from build123d import *

# Parameters (mm, degrees)
SKETCH1_R                           = 14.2875
SKETCH1_R_2                         = 9.525
BOSS_EXTRUDE1_DEPTH                 = 304.8
SKETCH2_R                           = 11.1125
CUT_EXTRUDE1_DEPTH                  = 19.05
CUT_EXTRUDE4_DEPTH                  = 76.2
CUT_EXTRUDE7_DEPTH                  = 12.7
CUT_EXTRUDE8_REACH                  = 308.326
CUT_EXTRUDE8_END_RADIUS             = 9.525
CUT_EXTRUDE8_DIRECTION_2_REACH      = 308.326
CUT_EXTRUDE8_DIRECTION_2_END_RADIUS = 14.2875


with BuildPart() as part:
    # Sketch1 → Boss-Extrude1 (new body)
    with BuildSketch(Plane.XY):
        with Locations(Location((0, 0, 0), (0, 0, 180))):
            Circle(SKETCH1_R)
        with Locations(Location((0, 0, 0), (0, 0, 180))):
            Circle(SKETCH1_R_2, mode=Mode.SUBTRACT)
    extrude(amount=BOSS_EXTRUDE1_DEPTH)

    # Sketch2 → Cut-Extrude1 (cut)
    with BuildSketch(Plane.XY.offset(304.8)):
        Circle(SKETCH2_R)
    extrude(amount=-CUT_EXTRUDE1_DEPTH, mode=Mode.SUBTRACT)

    # Sketch6 → Cut-Extrude4 (cut)
    with BuildSketch(Plane(origin=(0, 0, 0), x_dir=(-1, 0, 0), z_dir=(0, 0, -1))):
        with BuildLine():
            Line((14.2875, 0), (-14.2875, 0))
            ThreePointArc((-14.2875, 0), (0, -14.2875), (14.2875, 0))
        make_face()
    extrude(amount=-CUT_EXTRUDE4_DEPTH, mode=Mode.SUBTRACT)

    # Sketch8 → Cut-Extrude7 (cut)
    with BuildSketch(Plane(origin=(0, 0, 82.55), x_dir=(-1, 0, 0), z_dir=(0, 0, -1))):
        with BuildLine():
            ThreePointArc((-6.545430181, -12.7), (0, -14.2875), (6.545430181, -12.7))
            Line((6.545430181, -12.7), (-6.545430181, -12.7))
        make_face()
        with BuildLine():
            Line((-12.7, -6.545430181), (-12.7, 6.545430181))
            ThreePointArc((-12.7, 6.545430181), (-14.2875, 0), (-12.7, -6.545430181))
        make_face()
    extrude(amount=-CUT_EXTRUDE7_DEPTH, mode=Mode.SUBTRACT)

    # Cut-Extrude8: up to this cylinder (the profile starts outside it)
    cut_extrude8_end = Plane(origin=(0, 0, 171.45), z_dir=(0, 0, -1)) * Cylinder(CUT_EXTRUDE8_END_RADIUS, 636.702, mode=Mode.PRIVATE)
    # Sketch9 → Cut-Extrude8 (cut, up to the surface)
    with BuildSketch(Plane.XZ.offset(12.7), mode=Mode.PRIVATE) as cut_extrude8_sk1:
        with BuildLine():
            ThreePointArc((0, 174.625), (-3.175, 171.45), (0, 168.275))
            Line((0, 168.275), (0, 174.625))
        make_face()
    cut_extrude8_tool1 = extrude(cut_extrude8_sk1.sketch, amount=-CUT_EXTRUDE8_REACH, mode=Mode.PRIVATE) - cut_extrude8_end
    add(cut_extrude8_tool1.solids().sort_by_distance((-1.347512, -12.7, 171.45))[0], mode=Mode.SUBTRACT)
    # Sketch9 → Cut-Extrude8 (cut, up to the surface)
    with BuildSketch(Plane.XZ.offset(12.7), mode=Mode.PRIVATE) as cut_extrude8_sk2:
        with BuildLine():
            Line((0, 174.625), (0, 168.275))
            ThreePointArc((0, 168.275), (2.24506403, 169.20493597), (3.175, 171.45))
            ThreePointArc((3.175, 171.45), (2.24506403, 173.69506403), (0, 174.625))
        make_face()
    cut_extrude8_tool2 = extrude(cut_extrude8_sk2.sketch, amount=-CUT_EXTRUDE8_REACH, mode=Mode.PRIVATE) - cut_extrude8_end
    add(cut_extrude8_tool2.solids().sort_by_distance((1.347512, -12.7, 171.45))[0], mode=Mode.SUBTRACT)
    # Sketch9 → Cut-Extrude8 (cut, up to the surface)
    with BuildSketch(Plane.XZ.offset(12.7), mode=Mode.PRIVATE) as cut_extrude8_sk3:
        with BuildLine():
            ThreePointArc((0, 174.625), (-3.175, 171.45), (0, 168.275))
            Line((0, 168.275), (0, 174.625))
        make_face()
    cut_extrude8_tool3 = extrude(cut_extrude8_sk3.sketch, amount=-CUT_EXTRUDE8_REACH, mode=Mode.PRIVATE) - cut_extrude8_end
    add(cut_extrude8_tool3.solids().sort_by_distance((-1.347512, -12.7, 171.45))[0], mode=Mode.SUBTRACT)
    # Sketch9 → Cut-Extrude8 (cut, up to the surface)
    with BuildSketch(Plane.XZ.offset(12.7), mode=Mode.PRIVATE) as cut_extrude8_sk4:
        with BuildLine():
            Line((0, 174.625), (0, 168.275))
            ThreePointArc((0, 168.275), (2.24506403, 169.20493597), (3.175, 171.45))
            ThreePointArc((3.175, 171.45), (2.24506403, 173.69506403), (0, 174.625))
        make_face()
    cut_extrude8_tool4 = extrude(cut_extrude8_sk4.sketch, amount=-CUT_EXTRUDE8_REACH, mode=Mode.PRIVATE) - cut_extrude8_end
    add(cut_extrude8_tool4.solids().sort_by_distance((1.347512, -12.7, 171.45))[0], mode=Mode.SUBTRACT)

    # Cut-Extrude8 direction 2: up to this cylinder (the profile starts inside it)
    cut_extrude8_direction_2_end = Plane(origin=(0, 0, 171.45), z_dir=(0, 0, -1)) * Cylinder(CUT_EXTRUDE8_DIRECTION_2_END_RADIUS, 646.227, mode=Mode.PRIVATE)
    # Sketch9 → Cut-Extrude8 direction 2 (cut, up to the surface)
    with BuildSketch(Plane.XZ.offset(12.7), mode=Mode.PRIVATE) as cut_extrude8_direction_2_sk1:
        with BuildLine():
            ThreePointArc((0, 174.625), (-3.175, 171.45), (0, 168.275))
            Line((0, 168.275), (0, 174.625))
        make_face()
    cut_extrude8_direction_2_tool1 = extrude(cut_extrude8_direction_2_sk1.sketch, amount=CUT_EXTRUDE8_DIRECTION_2_REACH, mode=Mode.PRIVATE) & cut_extrude8_direction_2_end
    add(cut_extrude8_direction_2_tool1.solids().sort_by_distance((-1.347512, -12.7, 171.45))[0], mode=Mode.SUBTRACT)
    # Sketch9 → Cut-Extrude8 direction 2 (cut, up to the surface)
    with BuildSketch(Plane.XZ.offset(12.7), mode=Mode.PRIVATE) as cut_extrude8_direction_2_sk2:
        with BuildLine():
            Line((0, 174.625), (0, 168.275))
            ThreePointArc((0, 168.275), (2.24506403, 169.20493597), (3.175, 171.45))
            ThreePointArc((3.175, 171.45), (2.24506403, 173.69506403), (0, 174.625))
        make_face()
    cut_extrude8_direction_2_tool2 = extrude(cut_extrude8_direction_2_sk2.sketch, amount=CUT_EXTRUDE8_DIRECTION_2_REACH, mode=Mode.PRIVATE) & cut_extrude8_direction_2_end
    add(cut_extrude8_direction_2_tool2.solids().sort_by_distance((1.347512, -12.7, 171.45))[0], mode=Mode.SUBTRACT)
    # Sketch9 → Cut-Extrude8 direction 2 (cut, up to the surface)
    with BuildSketch(Plane.XZ.offset(12.7), mode=Mode.PRIVATE) as cut_extrude8_direction_2_sk3:
        with BuildLine():
            ThreePointArc((0, 174.625), (-3.175, 171.45), (0, 168.275))
            Line((0, 168.275), (0, 174.625))
        make_face()
    cut_extrude8_direction_2_tool3 = extrude(cut_extrude8_direction_2_sk3.sketch, amount=CUT_EXTRUDE8_DIRECTION_2_REACH, mode=Mode.PRIVATE) & cut_extrude8_direction_2_end
    add(cut_extrude8_direction_2_tool3.solids().sort_by_distance((-1.347512, -12.7, 171.45))[0], mode=Mode.SUBTRACT)
    # Sketch9 → Cut-Extrude8 direction 2 (cut, up to the surface)
    with BuildSketch(Plane.XZ.offset(12.7), mode=Mode.PRIVATE) as cut_extrude8_direction_2_sk4:
        with BuildLine():
            Line((0, 174.625), (0, 168.275))
            ThreePointArc((0, 168.275), (2.24506403, 169.20493597), (3.175, 171.45))
            ThreePointArc((3.175, 171.45), (2.24506403, 173.69506403), (0, 174.625))
        make_face()
    cut_extrude8_direction_2_tool4 = extrude(cut_extrude8_direction_2_sk4.sketch, amount=CUT_EXTRUDE8_DIRECTION_2_REACH, mode=Mode.PRIVATE) & cut_extrude8_direction_2_end
    add(cut_extrude8_direction_2_tool4.solids().sort_by_distance((1.347512, -12.7, 171.45))[0], mode=Mode.SUBTRACT)


solid = part.part
Verification items for the finished model (mm, model axes). A direction names the side the tool comes from. Coordinates: 2 decimals unless noted, no trailing zeros. Answer as a JSON object with one key per item and string values. Group by question number.
Item 1: Mould release check, pull along Y, two halves, no side actions. Record for faces 1 (the flat face through (0, 10, 0)), 2 (the cylindrical face through (3.097, 13.948, 150.266)), 3 (the cylindrical face through (10.6, 3.34, 295.41)), 4 (the cylindrical face through (-4.4, 8.45, 140.87)): +Y half, -Y half, draft (parallel to the pull), parting line (faces both ways), or undercut.
Item 2: Depth check by flat-ended pin: pin 1 (4 mm diameter, centred on x = 10.5, y = -6.5, fed in from -Z); pin 2 (1.4 mm diameter, centred on x = 12.5, z = 53.5, fed in from -Y); pin 3 (3 mm diameter, centred on y = 5.5, z = 189.5, fed in from -X). Enter the tip coordinate at first touch or a pass-through.
Item 3: Scan lines: probe 1 along X at (y, z) = (0.75, 120); probe 2 along Y at (x, z) = (0, 111) (1 decimal); probe 3 along Y at (x, z) = (0, 297.75). Record each from-to range of solid material in increasing order.
Item 4: Tool access check on faces 5 (the flat face through (12.7, 0, 89)), 6 (the flat face through (0, -12.7, 89)), 7 (the flat face through (-12, 0, 38)). Record the directions out of +Z, -Z, +X, -X, +Y, -Y that give a thin tool (end or side, any length) a straight path to the whole face; none if there is none.
Evaluation:
{
 "1": {"face 1": "draft", "face 2": "parting line", "face 3": "undercut", "face 4": "undercut"},
 "2": {"pin 1": "stops at z = 76.2", "pin 2": "stops at y = 0", "pin 3": "stops at x = -13.72"},
 "3": {"probe 1": "x = -14.27 to -9.5, 9.5 to 14.27", "probe 2": "y = -14.3 to -9.5, 9.5 to 14.3", "probe 3": "y = -14.29 to -11.11, 11.11 to 14.29"},
 "4": {"face 5": "+X, +Y, -Y", "face 6": "+X, -X, -Y", "face 7": "-Z, +X, -X, -Y"}
}
